Part model, mm, in its own coordinate system. Face numbers are marked on the shaded views. A direction names the side the tool comes from. Give positions to 0.01 mm unless a question says otherwise; leave off trailing zeros. Loops run counter-clockwise (first coordinate to the right, second up) from the corner with the lowest first, then second, coordinate; pieces in that order, holes last. Notation, with made-up numbers: M 53.5,84 L 62.5,84 A9 ccw 62.5,88 Z; hole C 26,-33 d3. An arc over 180 degrees is marked long. Put each result on its own line as item: value. Start each with the question number.
```python
from build123d import *

# Parameters (mm, degrees)
BOSS_EXTRU_1_DEPTH      = 10
ESQUISSE3_W             = 32
ESQUISSE3_H             = 5
BOSS_EXTRU_2_DEPTH      = 20
ESQUISSE4_R             = 2.5
BOSS_EXTRU_3_DEPTH      = 5
ESQUISSE6_R             = 1.7
ESQUISSE6_R_2           = 4
ESQUISSE6_R_3           = 1.6
ENL_V_MAT_EXTRU_1_DEPTH = 152.657508881


with BuildPart() as part:
    # Esquisse1 → Boss.-Extru.1 (new body)
    with BuildSketch(Plane.XY):
        with BuildLine():
            ThreePointArc((-16, 118), (0, 110), (16, 118))
            Line((16, 118), (16, 130))
            Line((16, 130), (-16, 130))
            Line((-16, 130), (-16, 118))
        make_face()
        with BuildLine():
            Line((16, 130), (16, 118))
            ThreePointArc((16, 118), (18.973665961, 123.67544468), (20, 130))
            ThreePointArc((20, 130), (-6.32455532, 148.973665961), (-16, 118))
            Line((-16, 118), (-16, 130))
            Line((-16, 130), (16, 130))
        make_face()
        with BuildLine():
            Line((-16, 0), (16, 0))
            Line((16, 0), (16, 118))
            ThreePointArc((16, 118), (0, 110), (-16, 118))
            Line((-16, 118), (-16, 0))
        make_face()
    extrude(amount=BOSS_EXTRU_1_DEPTH)

    # Esquisse3 → Boss.-Extru.2 (add)
    with BuildSketch(Plane.XZ):
        with Locations((0, 2.5)):
            Rectangle(ESQUISSE3_W, ESQUISSE3_H)
    extrude(amount=BOSS_EXTRU_2_DEPTH)

    # Esquisse4 → Boss.-Extru.3 (add)
    with BuildSketch(Plane.XY.offset(5)):
        with Locations(Location((-8, -10, 0), (0, 0, 180))):
            Circle(ESQUISSE4_R)
        with Locations(Location((8, -10, 0), (0, 0, 180))):
            Circle(ESQUISSE4_R)
    extrude(amount=BOSS_EXTRU_3_DEPTH)

    # Esquisse6 → Enlèv. mat.-Extru.1 (cut, through all)
    with BuildSketch(Plane.XY.offset(10)):
        with Locations((-6.717514421, 136.717514421)):
            Circle(ESQUISSE6_R)
        with Locations((6.717514421, 136.717514421)):
            Circle(ESQUISSE6_R)
        with Locations((6.717514421, 123.282485579)):
            Circle(ESQUISSE6_R)
        with Locations((-6.717514421, 123.282485579)):
            Circle(ESQUISSE6_R)
        with Locations((0, 75)):
            Circle(ESQUISSE6_R_2)
        with Locations((0, 2.83)):
            Circle(ESQUISSE6_R_3)
    extrude(amount=-ENL_V_MAT_EXTRU_1_DEPTH, mode=Mode.SUBTRACT)


solid = part.part
```
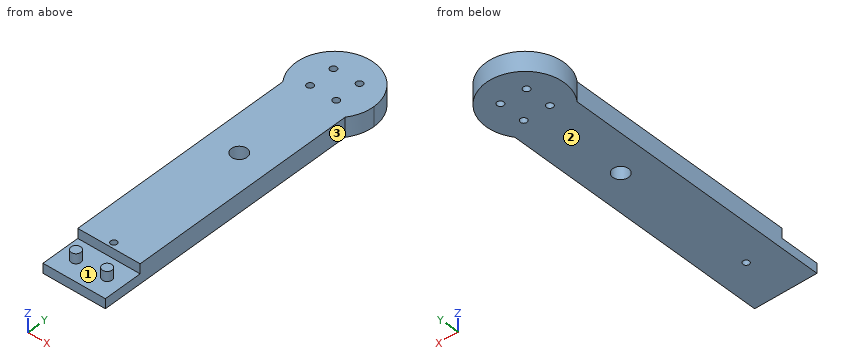
1) Wall check: L1, parallel to Y at x = 1, z = 5.25; L2, parallel to Y at x = -0.5, z = 0.5; L3, parallel to X at y = -7.5, z = 4.5. Give the ranges that are in metal, low to high.
2) Which spindle directions (+Z, -Z, +X, -X, +Y, -Y) get a long thin tool onto all of the face, cutting with end or side? Do the marked faces 1, 2 and 3. Say none if no direction does.
3) Band-saw the part on B-B on x = 0. Give the cut face in (y, z), then the cut area to 3 significant figures.
4) Band-saw the part on D-D on y = 2.83. Give the cut face in (x, z).
5) Band-saw the part on A-A on y = 75. Give the cut face in (x, z), then the cut area to 3 significant figures.
6) Band-saw the part on C-C on z = 8.5. State how many separate pieces and enclosed holes the cut face has, then the cut area to 3 significant figures.
7) Pin check, flat tips, straight feed: pin 1 Ø5 at (x, y) = (0, 75) entering from +Z; pin 2 Ø6 at (y, z) = (52.5, 8) entering from -X; pin 3 Ø1.5 at (x, z) = (-7, 7) entering from -Y; pin 4 Ø3 at (y, z) = (111, 2.5) entering from +X. Stop position of each tip, or through.
Evaluation:
1. L1: 0 to 1.58, 4.08 to 71.13, 78.87 to 149.97
1. L2: -20 to 1.31, 4.35 to 71.03, 78.97 to 149.99
1. L3: -16 to 16
2. face 1: +Z
2. face 2: -Z, +X, -X, +Y, -Y
2. face 3: +Z, -Z, +X, -Y
3. outline: M -20,0 L 1.23,0 L 1.23,10 L 0,10 L 0,5 L -20,5 Z; M 4.43,0 L 71,0 L 71,10 L 4.43,10 Z; M 79,0 L 150,0 L 150,10 L 79,10 Z
3. area: 1,490 mm2
4. outline: M -16,0 L -1.6,0 L -1.6,10 L -16,10 Z; M 1.6,0 L 16,0 L 16,10 L 1.6,10 Z
5. outline: M -16,0 L -4,0 L -4,10 L -16,10 Z; M 4,0 L 16,0 L 16,10 L 4,10 Z
5. area: 240 mm2
6. separate pieces: 3
6. enclosed holes: 6
6. area: 4,800 mm2
7. pin 1: through
7. pin 2: x = -16
7. pin 3: y = -12.49
7. pin 4: x = 16
